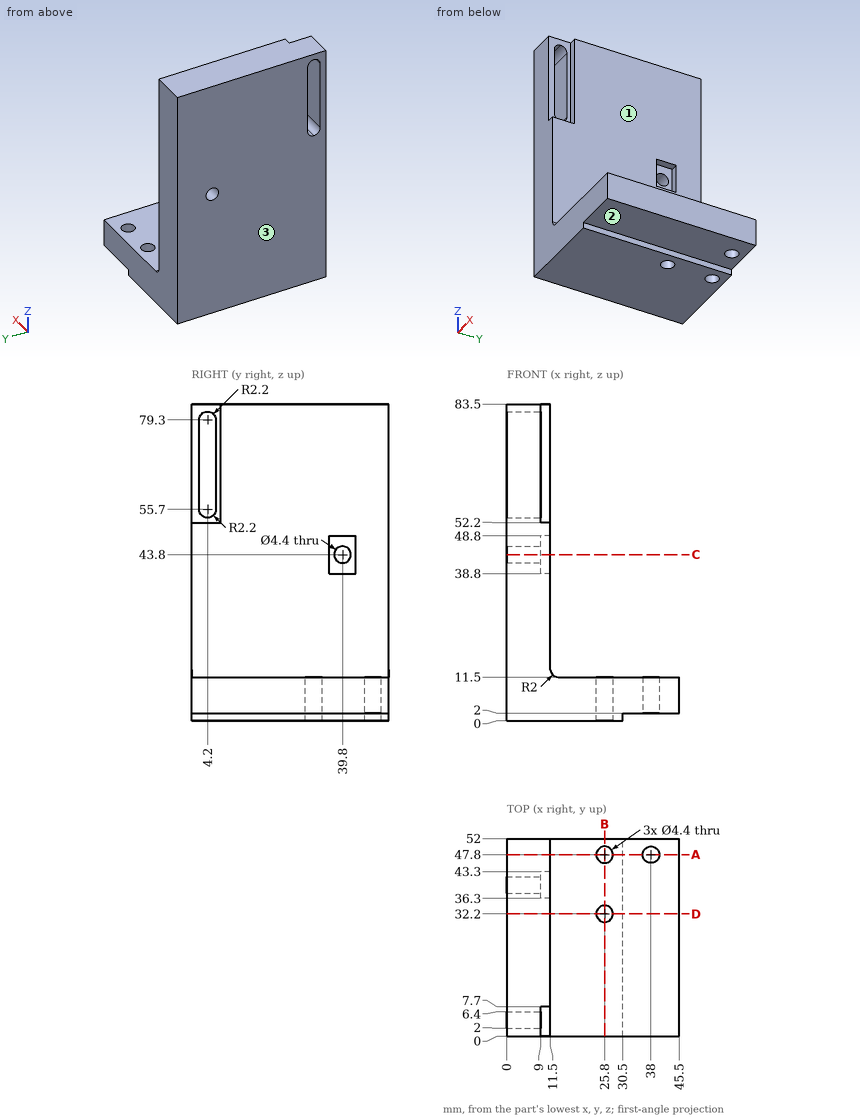
Could you check a few things on this drawing? It's one solid part, dimensions in mm from its lowest x, y, z. A direction names the side the tool comes from. Give positions to 0.01 mm unless a question says otherwise; leave off trailing zeros. Order: outer loops, then holes, each group sorted by start corner. A loop starts at its lowest first (then second) coordinate and runs counter-clockwise, first axis right, second up. Notation, with made-up numbers: (67.5, 74) - (91.5, 74) arc R17 cw to (91.5, 84) - close; hole circle Ø2 at (-16.5, 37.5). An arc over 180 degrees is marked (long way). One line per item, written item: value. Start each with the question number.
1. Imagine slicing it at B-B on x = 25.8. List the corners of the cut face in (y, z) for me.
2. Imagine slicing it at A-A on y = 47.8. List the corners of the cut face in (x, z) for me.
3. For P1, Ø1.2, axis at x = 10, y = 3.5, coming from the +Z side; P2, Ø7.5, axis at x = 35.5, y = 18.5, coming from the -Z side; P3, Ø3, axis at x = 38, y = 46.5, coming from the +Z side; P4, Ø1.5, axis at x = 13.5, z = 72, coming from the -Y side (1 decimal), each with a flat end and sliding along its axis, tell me the tip position at first contact or that it passes through.
4. For the marked faces 1, 2 and 3, which set-ups out of +Z, -Z, +X, -X, +Y, -Y let a thin tool reach every point of the face, with its end or its side?
5. Imagine slicing it at C-C on z = 43.8. List the corners of the cut face in (x, y) for me, plus the area to 3 significant figures.
6. Imagine slicing it at D-D on y = 32.2. List the corners of the cut face in (x, z) for me.
7. If I drill on probe 1 along Y at (x, z) = (25.8, 6); probe 2 along Y at (x, z) = (25, 6); probe 3 along Z at (x, y) = (31.5, 4), over which ranges is the centre line in solid material (lowest first)?
Values:
1. outline: (0, 0) - (30, 0) - (30, 11.5) - (0, 11.5) - close; (34.4, 0) - (45.6, 0) - (45.6, 11.5) - (34.4, 11.5) - close; (50, 0) - (52, 0) - (52, 11.5) - (50, 11.5) - close
2. outline: (0, 0) - (23.6, 0) - (23.6, 11.5) - (13.5, 11.5) arc R2 cw to (11.5, 13.5) - (11.5, 83.5) - (0, 83.5) - close; (28, 0) - (30.5, 0) - (30.5, 2) - (35.8, 2) - (35.8, 11.5) - (28, 11.5) - close; (40.2, 2) - (45.5, 2) - (45.5, 11.5) - (40.2, 11.5) - close
3. P1: z = 52.2
3. P2: z = 2
3. P3: z = 11.5
3. P4: through
4. face 1: +Z, +X, +Y, -Y
4. face 2: -Z, +X, +Y, -Y
4. face 3: +Z, -Z, -X, +Y, -Y
5. outline: (0, 0) - (11.5, 0) - (11.5, 36.3) - (9, 36.3) - (9, 37.6) - (0, 37.6) - close; (0, 42) - (9, 42) - (9, 43.3) - (11.5, 43.3) - (11.5, 52) - (0, 52) - close
5. area: 541 mm²
6. outline: (0, 0) - (23.6, 0) - (23.6, 11.5) - (13.5, 11.5) arc R2 cw to (11.5, 13.5) - (11.5, 83.5) - (0, 83.5) - close; (28, 0) - (30.5, 0) - (30.5, 2) - (45.5, 2) - (45.5, 11.5) - (28, 11.5) - close
7. probe 1: 0 to 30, 34.4 to 45.6, 50 to 52
7. probe 2: 0 to 30.15, 34.25 to 45.75, 49.85 to 52
7. probe 3: 2 to 11.5
